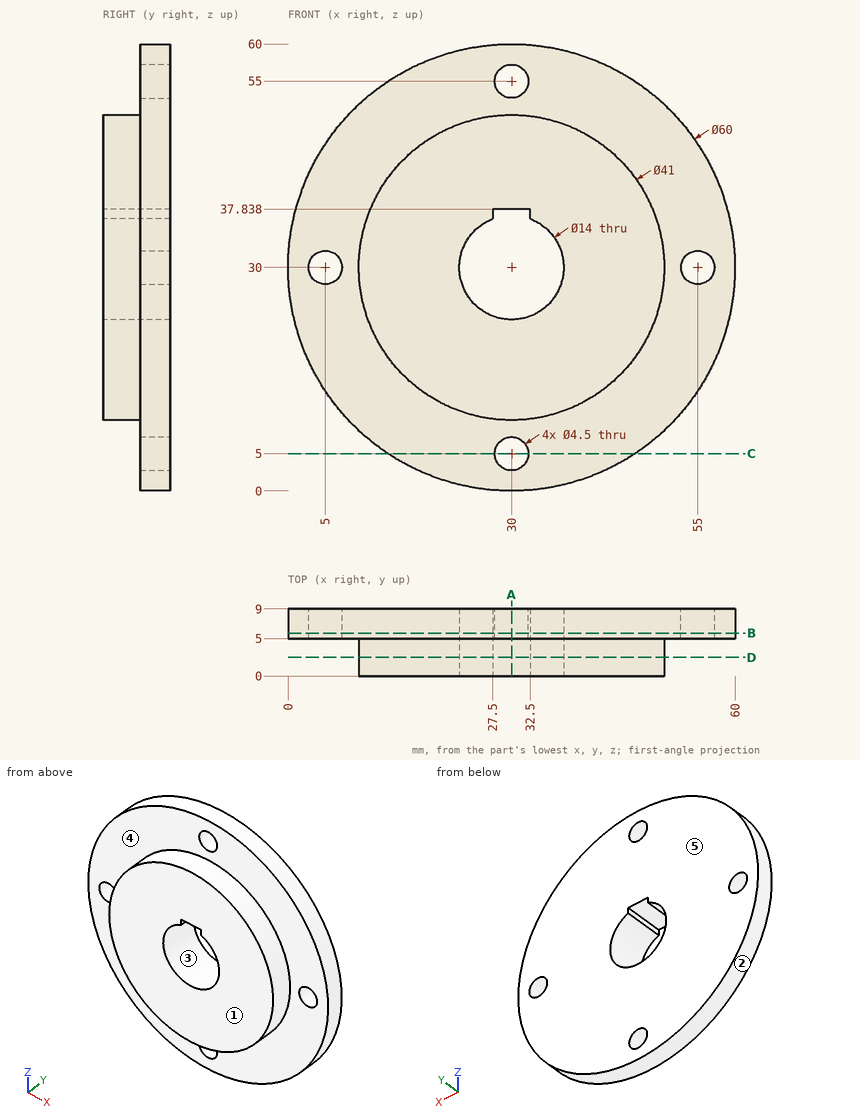
Part print with two shaded views. Sizes in mm from the minimum x, y, z corner. A direction names the side the tool comes from. Round coordinates to 2 decimals unless told otherwise and drop trailing zeros. Order: outer loops, then holes, each group sorted by start corner. A loop starts at its lowest first (then second) coordinate and runs counter-clockwise, first axis right, second up. Notation, with made-up numbers: (69.25, -8) - (87.25, -8) arc R33 cw to (87.25, 30) - close; hole circle Ø7 at (64.5, 50). An arc over 180 degrees is marked (long way). Answer as CSV lines item,"result". Start each with the question number.
1. Pull direction Z, two halves, no side cores. Call the marked faces 1, 2 and 3: +Z half, -Z half, draft (parallel to the pull), parting line (faces both ways), or undercut.
2. Saw through at B-B, the plane y = 5.75. Write the cut outline in (x, z).
3. Drill centre lines: L1, parallel to X at y = 5.85, z = 30; L2, parallel to Z at x = 35.5, y = 3.5; L3, parallel to Z at x = 33, y = 3 (1 decimal). Where is each one in solid material? Low to high. Write a range as [from, to].
4. Saw through at A-A, the plane x = 30. Write the cut outline in (y, z).
5. Pin check, flat tips, straight feed: pin 1 (5 mm diameter, centred on y = 8, z = 50, fed in from +X); pin 2 (2.5 mm diameter, centred on x = 55, z = 30, fed in from -Y); pin 3 (6 mm diameter, centred on x = 30, z = 55, fed in from -Y); pin 4 (1.5 mm diameter, centred on y = 4.5, z = 25, fed in from -X). Stop position of each tip, or through.
6. Saw through at C-C, the plane z = 5. Write the cut outline in (x, y), and give its area (3 significant figures).
7. Tool access for the marked faces 4 and 5: list every direction of +Z, -Z, +X, -X, +Y, -Y with a clear straight run to the whole face (end or side of a thin tool).
8. Saw through at D-D, the plane y = 2.5. Write the cut outline in (x, z).
Model answer:
1,face 1,"draft"
1,face 2,"parting line"
1,face 3,"undercut"
2,outline,"circle Ø60 at (30, 30); hole circle Ø4.5 at (5, 30); hole (27.5, 36.54) arc R7 ccw (long way) to (32.5, 36.54) - (32.5, 37.84) - (27.5, 37.84) - close; hole circle Ø4.5 at (30, 5); hole circle Ø4.5 at (30, 55); hole circle Ø4.5 at (55, 30)"
3,L1,"x = [0, 2.75], [7.25, 23], [37, 52.75], [57.25, 60]"
3,L2,"z = [10.25, 25.67], [34.33, 49.75]"
3,L3,"z = [9.7, 23.7], [36.3, 50.3]"
4,outline,"(0, 9.5) - (5, 9.5) - (5, 7.25) - (9, 7.25) - (9, 23) - (0, 23) - close; (0, 37.84) - (9, 37.84) - (9, 52.75) - (5, 52.75) - (5, 50.5) - (0, 50.5) - close; (5, 0) - (9, 0) - (9, 2.75) - (5, 2.75) - close; (5, 57.25) - (9, 57.25) - (9, 60) - (5, 60) - close"
5,pin 1,"stops at x = 54.37"
5,pin 2,"passes through"
5,pin 3,"stops at y = 5"
5,pin 4,"stops at x = 0.33"
6,outline,"(13.42, 5) - (27.75, 5) - (27.75, 9) - (13.42, 9) - close; (32.25, 5) - (46.58, 5) - (46.58, 9) - (32.25, 9) - close"
6,area,"115 mm²"
7,face 4,"-Y"
7,face 5,"+Z, -Z, +X, -X, +Y"
8,outline,"circle Ø41 at (30, 30); hole (27.5, 36.54) arc R7 ccw (long way) to (32.5, 36.54) - (32.5, 37.84) - (27.5, 37.84) - close"
